Answer from the drawing. Dimensions are ordinates in mm from the lowest x, y and z of the part. Coordinates: 2 decimals unless noted, no trailing zeros. Write each loop counter-clockwise with the first axis right and the second up, starting at its lowest first coordinate (ties: lowest second). Pieces come first, ordered by that corner, then holes.
(1) Determine the mould class of the marked faces 1, 2 and 3 for opening direction Z: pulls with the +Z half, pulls with the -Z half, needs draft (parallel to the pull), parting line crosses it, or undercut.
(2) Straight lines are drawn through the part: line 1 along Y through (x, z) = (5, 2.95); line 2 along Y through (x, z) = (6.25, 5.15); line 3 along X through (y, z) = (4.5, 2.25). For each, find the intervals that lie inside material, in ascending order.
(3) The part is cut by section B-B, the plane z = 2.9. Determine the outline of the cut face in (x, y).
(4) Given pin 1 (3 mm diameter, centred on x = 7, z = 3, fed in from -Y); pin 2 (1 mm diameter, centred on y = 6.5, z = 1.5, fed in from -X); pin 3 (2 mm diameter, centred on x = 3, z = 0.5, fed in from -Y); pin 4 (3 mm diameter, centred on x = 5, y = 5, fed in from -Z), each flat-ended and moving along its own axis, determine where each tip first touches the part or whether it passes through.
(5) The part is cut by section A-A, the plane x = 5. Determine the outline of the cut face in (y, z).
(6) The part is cut by section C-C, the plane z = 4.25. Determine the outline of the cut face in (x, y).
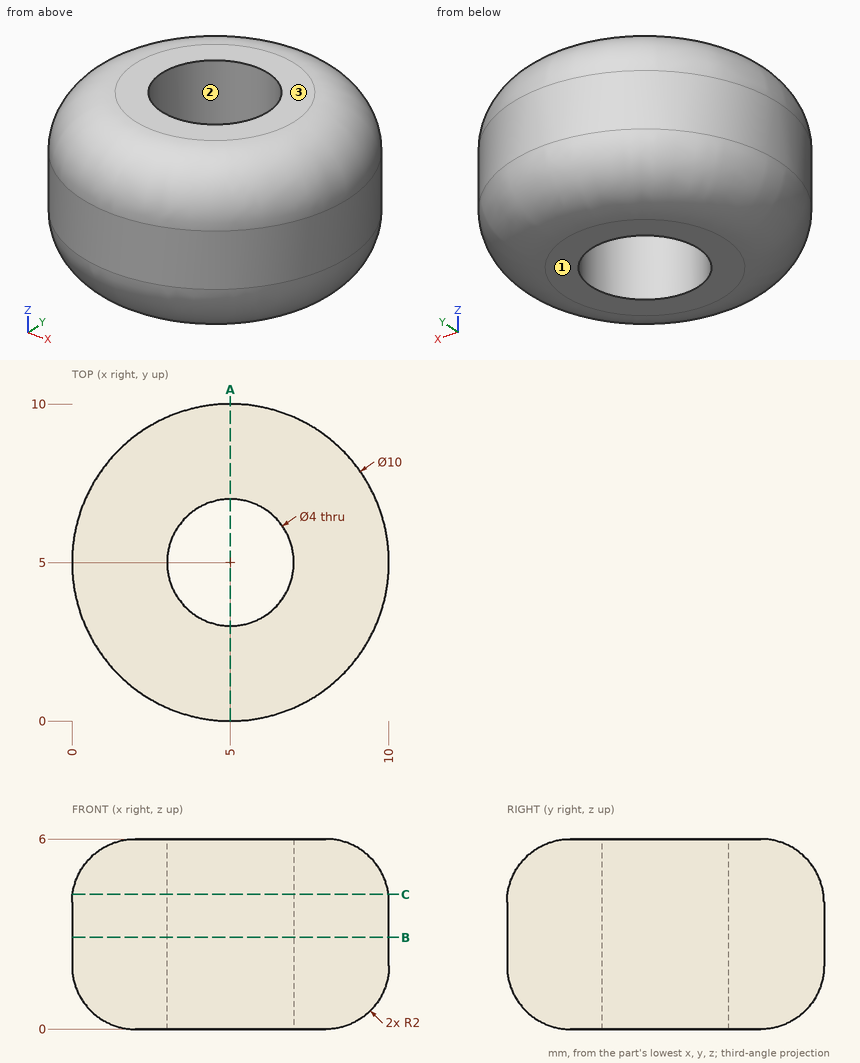
Computed:
1. face 1: pulls with the -Z half
1. face 2: needs draft
1. face 3: pulls with the +Z half
2. line 1: y = 0 to 3, 7 to 10
2. line 2: y = 0.54 to 3.44, 6.56 to 9.46
2. line 3: x = 0.03 to 3.06, 6.94 to 9.97
3. outline: circle Ø10 at (5, 5); hole circle Ø4 at (5, 5)
4. pin 1: stops at y = 0.03
4. pin 2: stops at x = 0.13
4. pin 3: stops at y = 0.33
4. pin 4: passes through
5. outline: (0, 2) arc R2 ccw to (2, 0) - (3, 0) - (3, 6) - (2, 6) arc R2 ccw to (0, 4) - close; (7, 0) - (8, 0) arc R2 ccw to (10, 2) - (10, 4) arc R2 ccw to (8, 6) - (7, 6) - close
6. outline: circle Ø9.97 at (5, 5); hole circle Ø4 at (5, 5)
